from build123d import *

# Parameters (mm, degrees)
SKETCH1_W           = 80
SKETCH1_H           = 50
BOSS_EXTRUDE1_DEPTH = 80
SHELL1_T            = -4
SKETCH2_W           = 76
SKETCH2_H           = 76
SKETCH2_W_2         = 72
SKETCH2_H_2         = 72
CUT_EXTRUDE1_DEPTH  = 20
SKETCH3_R           = 2.2
CUT_EXTRUDE2_DEPTH  = 124.693168769
FILLET1_R           = 0.5


with BuildPart() as part:
    # Sketch1 → Boss-Extrude1 (new body)
    with BuildSketch(Plane.XY):
        with Locations((40, 25)):
            Rectangle(SKETCH1_W, SKETCH1_H)
    extrude(amount=BOSS_EXTRUDE1_DEPTH)

    # Shell1
    shell1_openings = [part.faces().sort_by_distance(p)[0] for p in [
        (40, 50, 40),
    ]]
    offset(amount=SHELL1_T, openings=shell1_openings, kind=Kind.INTERSECTION)

    # Sketch2 → Cut-Extrude1 (cut)
    with BuildSketch(Plane(origin=(0, 50, 0), x_dir=(1, 0, 0), z_dir=(0, 1, 0))):
        with Locations((40, -40)):
            Rectangle(SKETCH2_W, SKETCH2_H)
        with Locations((40, -40)):
            Rectangle(SKETCH2_W_2, SKETCH2_H_2, mode=Mode.SUBTRACT)
    extrude(amount=-CUT_EXTRUDE1_DEPTH, mode=Mode.SUBTRACT)

    # Sketch3 → Cut-Extrude2 (cut, through all)
    with BuildSketch(Plane.XY.offset(80)):
        with Locations((20, 45)):
            Circle(SKETCH3_R)
        with Locations((60, 45)):
            Circle(SKETCH3_R)
    extrude(amount=-CUT_EXTRUDE2_DEPTH, mode=Mode.SUBTRACT)

    # Fillet1
    fillet1_edges = [part.edges().sort_by_distance(p)[0] for p in [
        (80, 25, 80),
        (40, 50, 80),
        (4, 30, 40),
        (40, 30, 76),
        (76, 30, 40),
        (40, 50, 2),
        (78, 50, 40),
        (40, 30, 78),
        (2, 30, 40),
        (40, 30, 4),
        (40, 30, 2),
        (78, 30, 40),
        (2, 50, 40),
        (40, 50, 78),
        (0, 25, 80),
        (40, 50, 0),
        (80, 25, 0),
        (40, 0, 0),
        (0, 25, 0),
        (0, 50, 40),
        (80, 50, 40),
        (80, 0, 40),
        (0, 0, 40),
        (40, 0, 80),
    ]]
    fillet(fillet1_edges, radius=FILLET1_R)


solid = part.part
The listing builds one solid part. Answer for the finished solid, in the listing's coordinates (mm). A direction names the side the tool comes from. Round coordinates to 2 decimals unless told otherwise and drop trailing zeros. Order: outer loops, then holes, each group sorted by start corner. A loop starts at its lowest first (then second) coordinate and runs counter-clockwise, first axis right, second up. Notation, with made-up numbers: (70.25, 42.5) - (97.25, 42.5) arc R12 cw to (97.25, 62.5) - close; hole circle Ø8 at (86.25, 70.25). An arc over 180 degrees is marked (long way). Write item = value, one per line. Start each with the question number.
1) Section A-A, the plane y = 35 is taken. Write down the section's boundary in (x, z), plus the area to 3 significant figures.
2) Section B-B, the plane x = 20 is taken. Count the separate pieces of the cut face and the enclosed holes in it, plus the area to 3 significant figures.
3) Straight lines are drawn through the part: L1, parallel to X at y = 22.5, z = 55.5; L2, parallel to Y at x = 60, z = 1.2; L3, parallel to Z at x = 74, y = 41.5. For each, find the intervals that lie inside material, in ascending order.
4) Section C-C, the plane y = 45 is taken. Write down the section's boundary in (x, z), plus the area to 3 significant figures.
5) Given pin 1 (5 mm diameter, centred on x = 60, y = 45, fed in from -Z); pin 2 (3 mm diameter, centred on x = 65, z = 13.5, fed in from +Y), each flat-ended and moving along its own axis, determine where each tip first touches the part or whether it passes through.
6) For faces 1 (the flat face through (39, 4, 39)), 2 (the cylindrical face through (61.02, 43.05, 79.01)), determine the directions among +Z, -Z, +X, -X, +Y, -Y from which every point of the face is accessible in a straight line to the end or side of a thin tool.
7) Section D-D, the plane z = 28 is taken. Write down the section's boundary in (x, y), plus the area to 3 significant figures.
8) For a pull along X with two mould halves and no side action, classify faces 3 (the flat face through (0, 25, 39)), 4 (the flat face through (39, 17, 4)), 5 (the flat face through (39, 25, 0)) as released by +X, released by -X, zero draft, split by the parting line, or undercut.
Results list:
q1.outline = (0, 0.5) arc R0.5 ccw to (0.5, 0) - (79.5, 0) arc R0.5 ccw to (80, 0.5) - (80, 79.5) arc R0.5 ccw to (79.5, 80) - (0.5, 80) arc R0.5 ccw to (0, 79.5) - close; hole (2, 2) - (78, 2) - (78, 78) - (2, 78) - close
q1.area = 624 mm^2
q2.separate_pieces = 3
q2.enclosed_holes = 0
q2.area = 590 mm^2
q3.L1 = 0 to 4, 76 to 80
q3.L2 = 0 to 42.8, 47.2 to 50
q3.L3 = 0 to 2, 78 to 80
q4.outline = (0, 0.5) arc R0.5 ccw to (0.5, 0) - (17.8, 0) - (17.8, 2) - (2, 2) - (2, 78) - (17.8, 78) - (17.8, 80) - (0.5, 80) arc R0.5 ccw to (0, 79.5) - close; (22.2, 0) - (57.8, 0) - (57.8, 2) - (22.2, 2) - close; (22.2, 78) - (57.8, 78) - (57.8, 80) - (22.2, 80) - close; (62.2, 0) - (79.5, 0) arc R0.5 ccw to (80, 0.5) - (80, 79.5) arc R0.5 ccw to (79.5, 80) - (62.2, 80) - (62.2, 78) - (78, 78) - (78, 2) - (62.2, 2) - close
q4.area = 589 mm^2
q5.pin_1 = 0
q5.pin_2 = 4
q6.face_1 = +Y
q6.face_2 = +Z, -Z
q7.outline = (0, 0.5) arc R0.5 ccw to (0.5, 0) - (79.5, 0) arc R0.5 ccw to (80, 0.5) - (80, 49.5) arc R0.5 ccw to (79.5, 50) - (78.5, 50) arc R0.5 ccw to (78, 49.5) - (78, 30.5) arc R0.5 cw to (77.5, 30) - (76.5, 30) arc R0.5 ccw to (76, 29.5) - (76, 4) - (4, 4) - (4, 29.5) arc R0.5 ccw to (3.5, 30) - (2.5, 30) arc R0.5 cw to (2, 30.5) - (2, 49.5) arc R0.5 ccw to (1.5, 50) - (0.5, 50) arc R0.5 ccw to (0, 49.5) - close
q7.area = 608 mm^2
q8.face_3 = released by -X
q8.face_4 = undercut
q8.face_5 = zero draft
